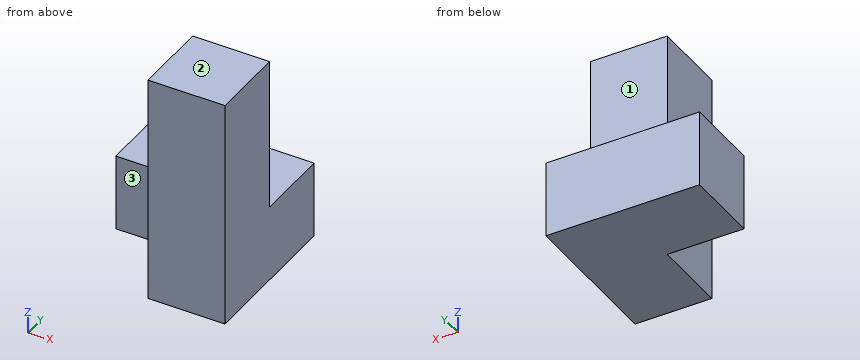
from build123d import *

# Parameters (mm, degrees)
F1_W     = 76.2
F1_H     = 76.2
F2_DEPTH = 228.6
F3_W     = 76.2
F3_H     = 76.2
F4_DEPTH = 76.2
F5_W     = 76.2
F5_H     = 76.2
F6_DEPTH = 76.2


# Not quite as in the source:
# - a variable given as a bare number and used for a length is read in inches; the dataset says mm whatever the document's units were


with BuildPart() as f2:
    # F1 (on Top) → F2 (new body)
    with BuildSketch(Plane.XY):
        Rectangle(F1_W, F1_H)
    extrude(amount=F2_DEPTH)

    # F3 (on face) → F4 (join)
    with BuildSketch(Plane(origin=(0, 38.1, 0), x_dir=(-1, 0, 0), z_dir=(0, 1, 0))):
        with Locations((0, 38.1)):
            Rectangle(F3_W, F3_H)
    extrude(amount=F4_DEPTH)

    # F5 (on face) → F6 (join)
    with BuildSketch(Plane(origin=(-38.1, 0, 0), x_dir=(0, -1, 0), z_dir=(-1, 0, 0))):
        with Locations((-76.2, 38.1)):
            Rectangle(F5_W, F5_H)
    extrude(amount=F6_DEPTH)


solid = f2.part
Could you check a few things on this model? Use its own coordinates, in mm. Face numbers are marked on the shaded views. A direction names the side the tool comes from. Coordinates: 2 decimals unless noted, no trailing zeros. Order: outer loops, then holes, each group sorted by start corner. A loop starts at its lowest first (then second) coordinate and runs counter-clockwise, first axis right, second up.
Q1. Suppose I cut it at A-A on x = 10. Please give me the cut outline in (y, z), and give its area (3 significant figures).
Q2. Suppose I cut it at B-B on z = 56.5. Please give me the cut outline in (x, y).
Q3. Which directions (+Z, -Z, +X, -X, +Y, -Y) give clear straight access to the entire face, cutting with the end or side of a thin tool? Please do the marked faces 1, 2 and 3.
Q4. Suppose I cut it at C-C on y = -10. Please give me the cut outline in (x, z), and give its area (3 significant figures).
Q5. Will these pins go through, and if not, where does the flat tip stop? pin 1 (2 mm diameter, centred on x = -39.5, y = 22.5, fed in from +Z); pin 2 (1 mm diameter, centred on y = -21, z = 45.5, fed in from -X); pin 3 (4 mm diameter, centred on x = -34, y = 88.5, fed in from +Z).
Q6. Please list where these lines run through material, in increasing order: L1, parallel to Y at x = -86, z = 23; L2, parallel to Y at x = -26.5, z = 121.5.
Q7. Suppose I cut it at D-D on z = 205. Please give me the cut outline in (x, y).
Answer:
1. outline: (-38.1, 0) - (114.3, 0) - (114.3, 76.2) - (38.1, 76.2) - (38.1, 228.6) - (-38.1, 228.6) - close
1. area: 23,200 mm2
2. outline: (-114.3, 38.1) - (-38.1, 38.1) - (-38.1, -38.1) - (38.1, -38.1) - (38.1, 114.3) - (-114.3, 114.3) - close
3. face 1: +Z, +X, -X, +Y
3. face 2: +Z, +X, -X, +Y, -Y
3. face 3: +Z, -Z, -X, -Y
4. outline: (-38.1, 0) - (38.1, 0) - (38.1, 228.6) - (-38.1, 228.6) - close
4. area: 17,400 mm2
5. pin 1: passes through
5. pin 2: stops at x = -38.1
5. pin 3: stops at z = 76.2
6. L1: y = 38.1 to 114.3
6. L2: y = -38.1 to 38.1
7. outline: (-38.1, -38.1) - (38.1, -38.1) - (38.1, 38.1) - (-38.1, 38.1) - close
